Work out the finished part from the listing and answer in its coordinate system (mm). Face numbers are marked on the shaded views. A direction names the side the tool comes from. Round coordinates to 2 decimals unless told otherwise and drop trailing zeros. Loops run counter-clockwise (first coordinate to the right, second up) from the corner with the lowest first, then second, coordinate; pieces in that order, holes last. Notation, with made-up numbers: (69.25, 61.5) - (98.25, 61.5) arc R21 cw to (98.25, 70.5) - close; hole circle Ø2 at (68.25, -29). An arc over 180 degrees is marked (long way). Use CSV: the item, a comma, the result in double quotes. Start each with the question number.
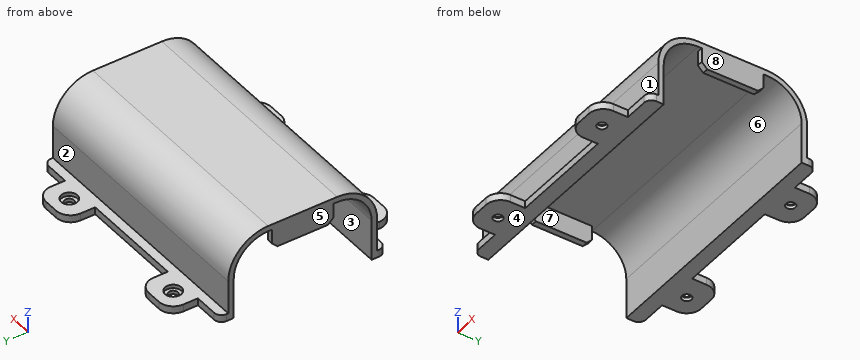
from build123d import *

# Parameters (mm, degrees)
PAD_DEPTH           = 70
POCKET_DEPTH        = 2.001
SKETCH002_R         = 1.3
POCKET001_DEPTH     = 2.001
SKETCH003_R         = 2.25
POCKET002_DEPTH     = 1
PAD001_DEPTH        = 1.6
LINEARPATTERN_COUNT = 2
LINEARPATTERN_PITCH = 68.4
FILLET_R            = 2
FILLET001_R         = 4
FILLET002_R         = 4


with BuildPart() as part:
    # Sketch → Pad (new body)
    with BuildSketch(Plane.YZ):
        with BuildLine():
            ThreePointArc((19, 11.2), (16.217514, 17.917514), (9.5, 20.7))
            Line((-9.5, 20.7), (9.5, 20.7))
            ThreePointArc((-9.5, 20.7), (-16.217514, 17.917514), (-19, 11.2))
            Line((-19, 11.2), (-19, 0))
            Line((-19, 0), (-31, 0))
            Line((-31, 0), (-31, 2))
            Line((-31, 2), (-20.5, 2))
            Line((-20.5, 2), (-20.5, 11.2))
            ThreePointArc((-9.5, 22.2), (-17.278175, 18.978175), (-20.5, 11.2))
            Line((-9.5, 22.2), (9.5, 22.2))
            ThreePointArc((20.5, 11.2), (17.278175, 18.978175), (9.5, 22.2))
            Line((20.5, 2), (20.5, 11.2))
            Line((31, 2), (20.5, 2))
            Line((31, 0), (31, 2))
            Line((19, 0), (31, 0))
            Line((19, 11.2), (19, 0))
        make_face()
    extrude(amount=PAD_DEPTH)

    # Sketch001 (on Face13 of Pad) → Pocket (cut, through all)
    with BuildSketch(Plane(origin=(0, 0, 2), x_dir=(0, -1, 0), z_dir=(0, 0, 1))):
        Polygon((23, 73), (23, 61.5), (35, 61.5), (35, 49.5), (23, 49.5), (23, 20.5), (35, 20.5), (35, 8.5), (23, 8.5), (23, -3), (46, -3), (46, 73), align=None)
        Polygon((-46, 73), (-23, 73), (-23, 61.5), (-35, 61.5), (-35, 49.5), (-23, 49.5), (-23, 20.5), (-35, 20.5), (-35, 8.5), (-23, 8.5), (-23, -3), (-46, -3), align=None)
    extrude(amount=-POCKET_DEPTH, mode=Mode.SUBTRACT)

    # Sketch002 (on Face17 of Pocket) → Pocket001 (cut, through all)
    with BuildSketch(Plane(origin=(0, 0, 2), x_dir=(0, -1, 0), z_dir=(0, 0, 1))):
        with Locations((26, 14)):
            Circle(SKETCH002_R)
        with Locations((-26, 14)):
            Circle(SKETCH002_R)
        with Locations((26, 55.5)):
            Circle(SKETCH002_R)
        with Locations((-26, 55.5)):
            Circle(SKETCH002_R)
    extrude(amount=-POCKET001_DEPTH, mode=Mode.SUBTRACT)

    # Sketch003 (on Face17 of Pocket001) → Pocket002 (cut)
    with BuildSketch(Plane(origin=(0, 0, 2), x_dir=(0, -1, 0), z_dir=(0, 0, 1))):
        with Locations((26, 55.5)):
            Circle(SKETCH003_R)
        with Locations((26, 14)):
            Circle(SKETCH003_R)
        with Locations((-26, 55.5)):
            Circle(SKETCH003_R)
        with Locations((-26, 14)):
            Circle(SKETCH003_R)
    extrude(amount=-POCKET002_DEPTH, mode=Mode.SUBTRACT)

    # Sketch004 → Pad001 (join)
    with BuildSketch(Plane.YZ):
        Polygon((-8.5, 21.3), (8.5, 21.3), (8.5, 16.8), (7, 15.3), (-7, 15.3), (-8.5, 16.8), align=None)
    pad001 = extrude(amount=PAD001_DEPTH)

    # LinearPattern: Pad001 ×2
    with Locations(*[(i * LINEARPATTERN_PITCH, 0, 0) for i in range(1, LINEARPATTERN_COUNT)]):
        add(pad001)

    # Fillet
    fillet_edges = [part.edges().sort_by_distance(p)[0] for p in [
        (70, 23, 1),
        (70, -23, 1),
        (0, -23, 1),
        (0, 23, 1),
    ]]
    fillet(fillet_edges, radius=FILLET_R)

    # Fillet001
    fillet001_edges = [part.edges().sort_by_distance(p)[0] for p in [
        (8.5, -31, 1),
        (20.5, -31, 1),
        (49.5, -31, 1),
        (61.5, -31, 1),
    ]]
    fillet(fillet001_edges, radius=FILLET001_R)

    # Fillet002
    fillet002_edges = [part.edges().sort_by_distance(p)[0] for p in [
        (61.5, 31, 1),
        (49.5, 31, 1),
        (20.5, 31, 1),
        (8.5, 31, 1),
    ]]
    fillet(fillet002_edges, radius=FILLET002_R)


solid = part.part
Item 1: The mould has two halves that part along X. Classify the marked faces 6, 7 and 8: pulls with the +X half, pulls with the -X half, needs draft (parallel to the pull), parting line crosses it, or undercut.
Item 2: A cutting plane is placed at A-A (y = 26). Determine the outline of the cut face in (x, z), plus the area to 3 significant figures.
Item 3: Find the intervals of material crossed by probe 1 along X at (y, z) = (26, 1.65); probe 2 along X at (y, z) = (-26, 0.4); probe 3 along X at (y, z) = (6, 16.5), in increasing order. Write a range as [from, to].
Item 4: Which of the six approach directions +Z, -Z, +X, -X, +Y, -Y give full straight-line access (tool end or side, diameter ignored) to the marked faces 1, 2, 3, 4 and 5?
Item 5: A cutting plane is placed at D-D (x = 39). Determine the outline of the cut face in (y, z), plus the area to 3 significant figures.
Item 6: A cutting plane is placed at B-B (z = 3.5). Determine the outline of the cut face in (x, y).
Item 7: A cutting plane is placed at C-C (x = 55.5). State how many separate pieces and enclosed holes the cut face has, plus the area to 3 significant figures.
Item 8: Each of these flat-tipped pins is pushed along its axis until it touches: pin 1 Ø1.6 at (x, z) = (64.5, 1) entering from +Y; pin 2 Ø12 at (x, z) = (21, 19) entering from -Y; pin 3 Ø0.5 at (x, z) = (69, 19.5) entering from -Y; pin 4 Ø8 at (y, z) = (-10.5, 11) entering from +X. Where does it stop, or does it pass through?
Result sheet:
1,face 6,"needs draft"
1,face 7,"undercut"
1,face 8,"pulls with the +X half"
2,outline,"(8.5, 0) - (12.7, 0) - (12.7, 1) - (11.75, 1) - (11.75, 2) - (8.5, 2) - close; (15.3, 0) - (20.5, 0) - (20.5, 2) - (16.25, 2) - (16.25, 1) - (15.3, 1) - close; (49.5, 0) - (54.2, 0) - (54.2, 1) - (53.25, 1) - (53.25, 2) - (49.5, 2) - close; (56.8, 0) - (61.5, 0) - (61.5, 2) - (57.75, 2) - (57.75, 1) - (56.8, 1) - close"
2,area,"33.8 mm^2"
3,probe 1,"[8.5, 11.75], [16.25, 20.5], [49.5, 53.25], [57.75, 61.5]"
3,probe 2,"[8.5, 12.7], [15.3, 20.5], [49.5, 54.2], [56.8, 61.5]"
3,probe 3,"[0, 1.6], [68.4, 70]"
4,face 1,"+Z, +X, -X, -Y"
4,face 2,"+Z, +X, -X, +Y"
4,face 3,"-Z, +X, -X"
4,face 4,"-Z, +X, -X, +Y, -Y"
4,face 5,"+Z, -Z, -X, +Y, -Y"
5,outline,"(-23, 0) - (-19, 0) - (-19, 11.2) arc R9.5 cw to (-9.5, 20.7) - (9.5, 20.7) arc R9.5 cw to (19, 11.2) - (19, 0) - (23, 0) - (23, 2) - (20.5, 2) - (20.5, 11.2) arc R11 ccw to (9.5, 22.2) - (-9.5, 22.2) arc R11 ccw to (-20.5, 11.2) - (-20.5, 2) - (-23, 2) - close"
5,area,"120 mm^2"
6,outline,"(0, -20.5) - (70, -20.5) - (70, -19) - (0, -19) - close; (0, 19) - (70, 19) - (70, 20.5) - (0, 20.5) - close"
7,separate pieces,"3"
7,enclosed holes,"0"
7,area,"138 mm^2"
8,pin 1,"y = 23"
8,pin 2,"y = -20.35"
8,pin 3,"y = -17"
8,pin 4,"through"
